from build123d import *

# Parameters (mm, degrees)
F0_W     = 114.3
F0_H     = 191.516
F1_DEPTH = 5.842
F2_W     = 5.842
F2_H     = 25.4
F2_W_2   = 25.4
F2_H_2   = 5.842
F3_DEPTH = 5.842
F5_DEPTH = 5.842


# Not quite as in the source:
# - a feature names something its author has since deleted; it is built from what else it names


with BuildPart() as f1:
    # F0 (on Front) → F1 (new body)
    with BuildSketch(Plane.XZ):
        with Locations((-13.1958257407, -66.1412229082)):
            Rectangle(F0_W, F0_H)
    extrude(amount=-F1_DEPTH)

    # F2 (on face) → F3 (cut, through all)
    with BuildSketch(Plane.XZ):
        with Locations((-67.4248257407, 4.2167770918)):
            Rectangle(F2_W, F2_H)
        with Locations((-67.4248257407, -136.4992229082)):
            Rectangle(F2_W, F2_H)
        with Locations((41.0331742593, 4.2167770918)):
            Rectangle(F2_W, F2_H)
        with Locations((-38.5958257407, 26.6957770918)):
            Rectangle(F2_W_2, F2_H_2)
        with Locations((12.2041742593, 26.6957770918)):
            Rectangle(F2_W_2, F2_H_2)
        Polygon((-70.3458257407, -75.1582229082), (-70.3458257407, -43.4082229082), (-79.5112612641, -43.4082229082), (-88.6766967875, -59.2832229082), (-79.5112612641, -75.1582229082), align=None)
        Polygon((-61.1803902173, -43.4082229082), (-70.3458257407, -43.4082229082), (-70.3458257407, -75.1582229082), (-61.1803902173, -75.1582229082), (-52.0149546939, -59.2832229082), align=None)
        Polygon((43.9541742593, -75.1582229082), (43.9541742593, -43.4082229082), (34.7887387359, -43.4082229082), (25.6233032125, -59.2832229082), (34.7887387359, -75.1582229082), align=None)
        Polygon((53.1196097827, -43.4082229082), (43.9541742593, -43.4082229082), (43.9541742593, -75.1582229082), (53.1196097827, -75.1582229082), (62.2850453061, -59.2832229082), align=None)
        Polygon((-26.0228257407, -142.8492229082), (-64.5038257407, -161.8992229082), (38.1121742593, -161.8992229082), (-0.3688257407, -142.8492229082), align=None)
        Polygon((-13.1958257407, -136.4992229082), (-26.0228257407, -142.8492229082), (-0.3688257407, -142.8492229082), align=None)
        Polygon((-38.5958257407, -142.8492229082), (-64.5038257407, -161.8992229082), (-26.0228257407, -142.8492229082), align=None)
        Polygon((-0.3688257407, -142.8492229082), (38.1121742593, -161.8992229082), (12.2041742593, -142.8492229082), align=None)
    extrude(amount=-F3_DEPTH, mode=Mode.SUBTRACT)

    # F4 (on face) → F5 (cut, through all)
    with BuildSketch(Plane.XZ):
        Polygon((5.1350453061, -59.2832229082), (-4.0303902173, -43.4082229082), (-22.3612612641, -43.4082229082), (-31.5266967875, -59.2832229082), (-22.3612612641, -75.1582229082), (-4.0303902173, -75.1582229082), align=None)
    extrude(amount=-F5_DEPTH, mode=Mode.SUBTRACT)


solid = f1.part
Check sheet for the modelled part. Datum: model origin and axes. Units: mm. A direction names the side the tool comes from. Round coordinates to 2 decimals unless told otherwise and drop trailing zeros. Order: outer loops, then holes, each group sorted by start corner. A loop starts at its lowest first (then second) coordinate and runs counter-clockwise, first axis right, second up.
(1) Access from +Z, -Z, +X, -X, +Y, -Y to the whole of each face (thin tool, end or side, straight path). Record for faces 5 (the flat face through (-39, 3, 23.775)), 6 (the flat face through (0.49, 2.88, -67.33)), 7 (the flat face through (-66, 3, -43.408)), 8 (the flat face through (-6.69, 2.88, -139.72)).
(2) Cross-section at D-D, the plane x = 14.5. Enter the section's corners in (y, z), and give its area (3 significant figures).
(3) Cross-section at A-A, the plane z = -68.5. Enter the section's corners in (x, y).
(4) Cross-section at B-B, the plane x = 2. Enter the section's corners in (y, z), and give its area (3 significant figures).
(5) Cross-section at C-C, the plane z = -5.5. Enter the section's corners in (x, y).
(6) Scan lines: probe 1 along Z at (x, y) = (39, 4.5); probe 2 along X at (y, z) = (4, -55); probe 3 along Z at (x, y) = (-29.5, 2.4). Record each from-to range of solid material in increasing order.
(7) Draft check along Z on faces 1 (the flat face through (43.954, 3, 23)), 2 (the flat face through (-64.504, 3, 4)), 3 (the flat face through (41, 3, -161.899)), 4 (the flat face through (-13, 3, 29.617)). Enter one of: pulls with the +Z half, pulls with the -Z half, needs draft (parallel to the pull), parting line crosses it, or undercut.
(8) Go/stop test with flat-tipped pins: P1, Ø1.8, axis at x = -34.5, y = 3.5, coming from the -Z side; P2, Ø2, axis at x = 5.5, y = 0.5, coming from the +Z side. Record where each tip stops, or that it passes through.
Check sheet entries:
1. face 5: +Z, +Y, -Y
1. face 6: +Y, -Y
1. face 7: -X, +Y, -Y
1. face 8: -Z, +Y, -Y
2. outline: (0, -144.54) - (5.84, -144.54) - (5.84, 23.77) - (0, 23.77) - close
2. area: 983 mm2
3. outline: (-57.34, 0) - (-26.21, 0) - (-26.21, 5.84) - (-57.34, 5.84) - close; (-0.19, 0) - (30.94, 0) - (30.94, 5.84) - (-0.19, 5.84) - close
4. outline: (0, -142.85) - (5.84, -142.85) - (5.84, -64.71) - (0, -64.71) - close; (0, -53.85) - (5.84, -53.85) - (5.84, 23.77) - (0, 23.77) - close
4. area: 910 mm2
5. outline: (-64.5, 0) - (38.11, 0) - (38.11, 5.84) - (-64.5, 5.84) - close
6. probe 1: z = -161.9 to -75.16, -43.41 to -8.48, 16.92 to 29.62
6. probe 2: x = -54.49 to -29.05, 2.66 to 28.1
6. probe 3: z = -142.85 to -62.79, -55.77 to 23.77
7. face 1: needs draft
7. face 2: undercut
7. face 3: pulls with the -Z half
7. face 4: pulls with the +Z half
8. P1: stops at z = -142.85
8. P2: stops at z = 23.77
